Verification items for the finished model (mm, model axes). A direction names the side the tool comes from. Coordinates: 2 decimals unless noted, no trailing zeros. Loops run counter-clockwise (first coordinate to the right, second up) from the corner with the lowest first, then second, coordinate; pieces in that order, holes last. Notation, with made-up numbers: M 32.5,27 L 54.5,27 A28 ccw 54.5,57 Z; hole C 75,12.5 d9. An arc over 180 degrees is marked long. Write item = value, one per line. Start each with the question number.
```python
from build123d import *

# Parameters (mm, degrees)
EXTRUSION4_DEPTH = 25.4


with BuildPart() as part:
    # Sketch1 → Extrusion4 (new body)
    with BuildSketch(Plane.XY):
        with BuildLine():
            Line((-14.999999544, 15.00000004), (-4.099998054, 15.00000004))
            Line((-4.099998054, 15.00000004), (-4.099998054, 12.50000004))
            Line((-4.099998054, 12.50000004), (-6.799995004, 12.50000004))
            Line((-6.799995004, 12.50000004), (-6.799995004, 7.86065564))
            Line((-6.799995004, 7.86065564), (-3.941497574, 5.00215821))
            Line((-3.941497574, 5.00215821), (3.941498416, 5.00215821))
            Line((3.941498416, 5.00215821), (6.799995846, 7.86065564))
            Line((6.799995846, 7.86065564), (6.799995846, 12.50000004))
            Line((6.799995846, 12.50000004), (4.099998896, 12.50000004))
            Line((4.099998896, 12.50000004), (4.099998896, 15.00000004))
            Line((4.099998896, 15.00000004), (15.000000416, 15.00000004))
            Line((15.000000416, 15.00000004), (15.000000416, 12.05771371))
            ThreePointArc((15.000000416, 12.05771371), (12.955549997, -3.471428997), (6.961524646, -17.94228629))
            Line((6.961524646, -17.94228629), (5.490381513, -20.490381017))
            Line((5.490381513, -20.490381017), (-3.949296731, -15.040380238))
            Line((-3.949296731, -15.040380238), (-2.699296736, -12.875316731))
            Line((-2.699296736, -12.875316731), (-0.361030787, -14.225315201))
            Line((-0.361030787, -14.225315201), (1.958641406, -10.2075251))
            Line((1.958641406, -10.2075251), (0.912358736, -6.302745))
            Line((0.912358736, -6.302745), (-5.914516044, -2.36124701))
            Line((-5.914516044, -2.36124701), (-9.819296144, -3.40752968))
            Line((-9.819296144, -3.40752968), (-12.138968342, -7.425319789))
            Line((-12.138968342, -7.425319789), (-9.800702394, -8.775318258))
            Line((-9.800702394, -8.775318258), (-11.050702387, -10.940381761))
            Line((-11.050702387, -10.940381761), (-20.490380619, -5.490380991))
            Line((-20.490380619, -5.490380991), (-19.019237434, -2.94228629))
            ThreePointArc((-19.019237434, -2.94228629), (-16.022224761, 4.293142357), (-14.999999544, 12.05771371))
            Line((-14.999999544, 12.05771371), (-14.999999544, 15.00000004))
        make_face()
        with BuildLine():
            Line((-3.499999544, 2.08578648), (-3.499999544, 3.00000004))
            ThreePointArc((-3.499999544, 3.00000004), (-3.353552934, 3.35355343), (-2.999999544, 3.50000004))
            Line((-2.999999544, 3.50000004), (-2.085785994, 3.50000006))
            Line((-2.085785994, 3.50000006), (-2.005133554, 3.41934762))
            ThreePointArc((-2.005133554, 3.41934762), (-1.841799553, 3.33547501), (-1.660186564, 3.36248117))
            ThreePointArc((-1.660186564, 3.36248117), (4.31e-07, 3.75000007), (1.660187426, 3.36248117))
            ThreePointArc((1.660187426, 3.36248117), (1.841800416, 3.33547501), (2.005134416, 3.41934762))
            Line((2.005134416, 3.41934762), (2.085786856, 3.50000006))
            Line((2.085786856, 3.50000006), (3.000000416, 3.50000006))
            ThreePointArc((3.000000416, 3.50000006), (3.353553806, 3.35355345), (3.500000416, 3.00000006))
            Line((3.500000416, 3.00000006), (3.500000416, 2.0857865))
            Line((3.500000416, 2.0857865), (3.419347976, 2.00513406))
            ThreePointArc((3.419347976, 2.00513406), (3.335475366, 1.841800059), (3.362481526, 1.66018707))
            ThreePointArc((3.362481526, 1.66018707), (3.622222275, -0.970571346), (2.081900986, -3.11900459))
            ThreePointArc((2.081900986, -3.11900459), (1.967706477, -3.262782979), (1.958675286, -3.44617068))
            Line((1.958675286, -3.44617068), (1.988196126, -3.55634396))
            Line((1.988196126, -3.55634396), (1.531089346, -4.34807613))
            ThreePointArc((1.531089346, -4.34807613), (1.227486167, -4.58103904), (0.848076646, -4.53108883))
            Line((0.848076646, -4.53108883), (0.056344476, -4.07398205))
            Line((0.056344476, -4.07398205), (0.026823636, -3.96380877))
            ThreePointArc((0.026823636, -3.96380877), (-0.072691445, -3.809505949), (-0.243475994, -3.74208748))
            ThreePointArc((-0.243475994, -3.74208748), (-1.874999553, -3.247595194), (-3.119004214, -2.08190049))
            ThreePointArc((-3.119004214, -2.08190049), (-3.262782603, -1.967705981), (-3.446170304, -1.95867479))
            Line((-3.446170304, -1.95867479), (-3.556343584, -1.98819563))
            Line((-3.556343584, -1.98819563), (-4.348075754, -1.53108885))
            ThreePointArc((-4.348075754, -1.53108885), (-4.581038663, -1.227485671), (-4.531088454, -0.84807615))
            Line((-4.531088454, -0.84807615), (-4.073981674, -0.05634398))
            Line((-4.073981674, -0.05634398), (-3.963808394, -0.02682314))
            ThreePointArc((-3.963808394, -0.02682314), (-3.809505572, 0.072691941), (-3.742087104, 0.24347649))
            ThreePointArc((-3.742087104, 0.24347649), (-3.622221403, 0.970571473), (-3.362480654, 1.66018705))
            ThreePointArc((-3.362480654, 1.66018705), (-3.335474493, 1.841800039), (-3.419347104, 2.00513404))
            Line((-3.419347104, 2.00513404), (-3.499999544, 2.08578648))
        make_face(mode=Mode.SUBTRACT)
        with BuildLine():
            Line((7.799995876, 7.56776241), (7.799995866, 14.00000004))
            Line((7.799995866, 14.00000004), (14.000000436, 14.00000004))
            Line((14.000000436, 14.00000004), (14.000000436, 12.05771371))
            ThreePointArc((14.000000436, 12.05771371), (13.543013967, 4.72862326), (12.179133767, -2.486931761))
            Line((12.179133767, -2.486931761), (5.615359986, -0.72817388))
            ThreePointArc((5.615359986, -0.72817388), (5.341691374, -0.541062306), (5.245224376, -0.22388827))
            ThreePointArc((5.245224376, -0.22388827), (5.222856323, 0.533175972), (5.091787186, 1.27914345))
            ThreePointArc((5.091787186, 1.27914345), (5.115773337, 3.319255981), (6.142816616, 5.08215603))
            Line((6.142816616, 5.08215603), (7.214209436, 6.15354885))
            ThreePointArc((7.214209436, 6.15354885), (7.647754936, 6.802395548), (7.799995876, 7.56776241))
        make_face(mode=Mode.SUBTRACT)
        with BuildLine():
            Line((5.227131414, -2.177062614), (11.790905183, -3.935820492))
            ThreePointArc((11.790905183, -3.935820492), (9.364282579, -10.866614542), (6.095499246, -17.44228629))
            Line((6.095499246, -17.44228629), (5.124356099, -19.124355612))
            Line((5.124356099, -19.124355612), (-0.245005373, -16.024353311))
            Line((-0.245005373, -16.024353311), (2.971113436, -10.45387213))
            ThreePointArc((2.971113436, -10.45387213), (3.221952356, -9.714924516), (3.170914286, -8.93623404))
            Line((3.170914286, -8.93623404), (2.778757296, -7.47268423))
            ThreePointArc((2.778757296, -7.47268423), (2.770761748, -5.432446365), (3.770045396, -3.65366401))
            ThreePointArc((3.770045396, -3.65366401), (4.256538339, -3.07317179), (4.654441766, -2.42871895))
            ThreePointArc((4.654441766, -2.42871895), (4.896571658, -2.202271683), (5.227131414, -2.177062614))
        make_face(mode=Mode.SUBTRACT)
        with BuildLine():
            Line((-13.999999544, 14.00000005), (-7.799994974, 14.00000005))
            Line((-7.799994974, 14.00000005), (-7.799994974, 7.56776243))
            ThreePointArc((-7.799994974, 7.56776243), (-7.647754043, 6.802395559), (-7.214208534, 6.15354886))
            Line((-7.214208534, 6.15354886), (-6.102918804, 5.04225913))
            ThreePointArc((-6.102918804, 5.04225913), (-5.119406434, 1.371740988), (-7.806412204, -1.31526478))
            Line((-7.806412204, -1.31526478), (-9.324462204, -1.72202505))
            ThreePointArc((-9.324462204, -1.72202505), (-10.024346973, -2.06717002), (-10.538874924, -2.6538767))
            Line((-10.538874924, -2.6538767), (-13.754993733, -8.224357881))
            Line((-13.754993733, -8.224357881), (-19.124355202, -5.12435558))
            Line((-19.124355202, -5.12435558), (-18.153212024, -3.44228628))
            ThreePointArc((-18.153212024, -3.44228628), (-15.056298932, 4.034323322), (-13.999999544, 12.05771372))
            Line((-13.999999544, 12.05771372), (-13.999999544, 14.00000005))
        make_face(mode=Mode.SUBTRACT)
    extrude(amount=EXTRUSION4_DEPTH)


solid = part.part
```
Q1. Sectioned sample at D-D on z = 19.75. Count the separate pieces of the cut face and the enclosed holes in it, plus the area to 3 significant figures.
Q2. Gauge pin test, flat ends, axial feed: pin 1 (10 mm diameter, centred on y = 0, z = 21, fed in from -X); pin 2 (1.6 mm diameter, centred on y = 13, z = 15.5, fed in from -X); pin 3 (12 mm diameter, centred on x = 11, z = 7, fed in from -Y); pin 4 (1.3 mm diameter, centred on x = -5.5, z = 7.5, fed in from -Y). Record the tip position at first contact, or that the pin passes through.
Q3. Set-up check for faces 1 (the face through (0, 5.002, 13)), 2 (the face through (6.8, 10, 13)), 3 (the face through (-15, 14, 13)): record each of +Z, -Z, +X, -X, +Y, -Y from which the full face is reachable in a straight line by a thin tool's end or side.
Q4. Sectioned sample at A-A on x = -14.5. Record the cut outline in (y, z).
Q5. Mould release check, pull along Y, two halves, no side actions. Record for faces 4 (the face through (-16.05, 4.19, 12.52)), 5 (the face through (6.236, -19.198, 12.522)), 6 (the face through (4.25, -3.08, 12.52)): +Y half, -Y half, draft (parallel to the pull), parting line (faces both ways), or undercut.
Q6. Scan lines: L1, parallel to Y at x = 4.5, z = 14.5; L2, parallel to X at y = 4, z = 15.25; L3, parallel to X at y = 11, z = 9.5. Record each from-to range of solid material in increasing order. Write a range as [from, to].
Q7. Sectioned sample at C-C on x = -1. Record the cut outline in (y, z), plus the area to 3 significant figures.
Q8. Sectioned sample at B-B on y = 9. Record the cut outline in (x, z), plus the area to 3 significant figures.
Solutions:
q1.separate_pieces = 1
q1.enclosed_holes = 4
q1.area = 226 mm²
q2.pin_1 = -20.21
q2.pin_2 = -15
q2.pin_3 = -20.49
q2.pin_4 = -2.98
q3.face_1 = +Z, -Z, +Y
q3.face_2 = +Z, -Z
q3.face_3 = +Z, -Z, -X, +Y
q4.outline = M -8.95,0 L -7.79,0 L -7.79,25.4 L -8.95,25.4 Z; M 6.51,0 L 15,0 L 15,25.4 L 6.51,25.4 Z
q5.face_4 = +Y half
q5.face_5 = -Y half
q5.face_6 = undercut
q6.L1 = [-19.92, -18.76], [-2.7, 5.56], [12.5, 15]
q6.L2 = [-16.1, -15.07], [-5.36, 5.37], [13.45, 14.46]
q6.L3 = [-15.02, -14.02], [-7.8, -6.8], [6.8, 7.8], [13.99, 14.99]
q7.outline = M -16.74,0 L -13.86,0 L -13.86,25.4 L -16.74,25.4 Z; M -5.2,0 L -3.61,0 L -3.61,25.4 L -5.2,25.4 Z; M 3.61,0 L 5,0 L 5,25.4 L 3.61,25.4 Z
q7.area = 149 mm²
q8.outline = M -15.16,0 L -14.15,0 L -14.15,25.4 L -15.16,25.4 Z; M -7.8,0 L -6.8,0 L -6.8,25.4 L -7.8,25.4 Z; M 6.8,0 L 7.8,0 L 7.8,25.4 L 6.8,25.4 Z; M 13.92,0 L 14.92,0 L 14.92,25.4 L 13.92,25.4 Z
q8.area = 102 mm²
